Build history of the part. All positions in model axes, mm. Face numbers are marked on the shaded views. A direction names the side the tool comes from. Give positions to 0.01 mm unless a question says otherwise; leave off trailing zeros. Write each loop counter-clockwise with the first axis right and the second up, starting at its lowest first coordinate (ties: lowest second). Pieces come first, ordered by that corner, then holes. Notation, with made-up numbers: (80.25, 63) -> (99.25, 63) arc R22 cw to (99.25, 101) -> close; hole circle Ø1 at (38.25, -11.5). An arc over 180 degrees is marked (long way). Put each result on its own line as item: value.
from build123d import *

# Parameters (mm, degrees)
SKETCH_1_R          = 9
EXTRUDE_1_DEPTH     = 8
SKETCH_5_R          = 3
SKETCH_2_R          = 3
CUT_EXTRUDE_1_DEPTH = 16.033296378
SKETCH_6_R          = 4.25
CUT_EXTRUDE_2_DEPTH = 3


with BuildPart() as part:
    # 草图1 → 凸台-拉伸1 (new body)
    with BuildSketch(Plane(origin=(0, 0, 0), x_dir=(1, 0, 0), z_dir=(0, 1, 0))):
        with Locations(Location((0, 0, 0), (0, 0, 270))):
            Circle(SKETCH_1_R)
    extrude(amount=EXTRUDE_1_DEPTH)

    # 草图5 → 切除-旋转1 (revolve, cut)
    with BuildSketch(Plane(origin=(0, 0, 0), x_dir=(0, 0, -1), z_dir=(1, 0, 0)), mode=Mode.PRIVATE) as cut_revolve_1_sk:
        with Locations((9, 4)):
            Circle(SKETCH_5_R)
    revolve(cut_revolve_1_sk.sketch.rotate(Axis((0, 8, 0), (0, -1, 0)), 180), axis=Axis((0, 8, 0), (0, -1, 0)), mode=Mode.SUBTRACT)

    # 草图2 → 切除-拉伸1 (cut, through all)
    with BuildSketch(Plane(origin=(0, 8, 0), x_dir=(1, 0, 0), z_dir=(0, 1, 0))):
        with Locations(Location((0, 0, 0), (0, 0, 270))):
            Circle(SKETCH_2_R)
    extrude(amount=-CUT_EXTRUDE_1_DEPTH, mode=Mode.SUBTRACT)

    # 草图6 → 切除-拉伸2 (cut)
    with BuildSketch(Plane(origin=(0, 8, 0), x_dir=(1, 0, 0), z_dir=(0, 1, 0))):
        with Locations(Location((0, 0, 0), (0, 0, 270))):
            Circle(SKETCH_6_R)
    cut_extrude_2 = extrude(amount=-CUT_EXTRUDE_2_DEPTH, mode=Mode.SUBTRACT)

    # 镜向2: 切除-拉伸2 across plane
    add(cut_extrude_2.mirror(Plane(origin=(0, 4, 0), x_dir=(0, 0, 1), z_dir=(0, -1, 0))), mode=Mode.SUBTRACT)


solid = part.part
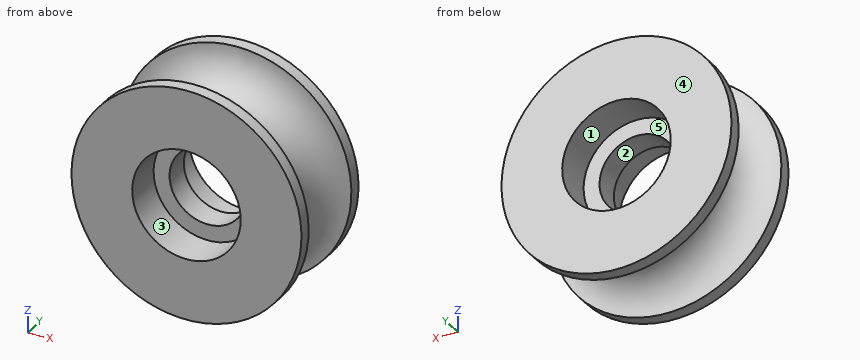
1) Slice it at B-B (z = 0). Write the cut outline in (x, y), plus the area to 3 significant figures.
Filled sheet:
outline: (-9, 0) -> (-4.25, 0) -> (-4.25, 3) -> (-3, 3) -> (-3, 5) -> (-4.25, 5) -> (-4.25, 8) -> (-9, 8) -> (-9, 7) arc R3 cw to (-9, 1) -> close; (3, 3) -> (4.25, 3) -> (4.25, 0) -> (9, 0) -> (9, 1) arc R3 cw to (9, 7) -> (9, 8) -> (4.25, 8) -> (4.25, 5) -> (3, 5) -> close
area: 52.7 mm2
2) Slice it at C-C (y = 4.75). Write the cut outline in (x, z).
Filled sheet:
outline: circle Ø12.19 at (0, 0); hole circle Ø6 at (0, 0)
3) Wall check: L1, parallel to X at y = 4.5, z = 2; L2, parallel to X at y = 6.4, z = 0; L3, parallel to Y at x = -3, z = 2.5. Give the ranges that are in metal, low to high.
Filled sheet:
L1: -5.7 to -2.24, 2.24 to 5.7
L2: -7.2 to -4.25, 4.25 to 7.2
L3: 3 to 5
4) Tool access for the marked faces 1, 2 and 3: list every direction of +Z, -Z, +X, -X, +Y, -Y with a clear straight run to the whole face (end or side of a thin tool).
Filled sheet:
face 1: +Y
face 2: +Y, -Y
face 3: -Y
5) Pull direction Z, two halves, no side cores. Call the marked faces 4 and 5: released by +Z, released by -Z, zero draft, split by the parting line, or undercut.
Filled sheet:
face 4: zero draft
face 5: undercut
6) Slice it at A-A (x = 0). Write the cut outline in (y, z), plus the area to 3 significant figures.
Filled sheet:
outline: (0, -9) -> (1, -9) arc R3 cw to (7, -9) -> (8, -9) -> (8, -4.25) -> (5, -4.25) -> (5, -3) -> (3, -3) -> (3, -4.25) -> (0, -4.25) -> close; (0, 4.25) -> (3, 4.25) -> (3, 3) -> (5, 3) -> (5, 4.25) -> (8, 4.25) -> (8, 9) -> (7, 9) arc R3 cw to (1, 9) -> (0, 9) -> close
area: 52.7 mm2
7) Pin check, flat tips, straight feed: pin 1 (1 mm diameter, centred on x = 3.5, y = 1, fed in from +Z); pin 2 (10 mm diameter, centred on x = 0, z = 0, fed in from -Y); pin 3 (7 mm diameter, centred on x = 0, z = 0, fed in from -Y). Stop position of each tip, or through.
Filled sheet:
pin 1: z = 8.49
pin 2: y = 0
pin 3: y = 3
